Part print with two shaded views. Sizes in mm from the minimum x, y, z corner. A direction names the side the tool comes from. Give positions to 0.01 mm unless a question says otherwise; leave off trailing zeros. Order: outer loops, then holes, each group sorted by start corner. A loop starts at its lowest first (then second) coordinate and runs counter-clockwise, first axis right, second up. Notation, with made-up numbers: M 1.5,31.5 L 20.5,31.5 A16 ccw 20.5,62.5 Z; hole C 47,41.25 d4. An arc over 180 degrees is marked long. Answer as CSV lines item,"result".
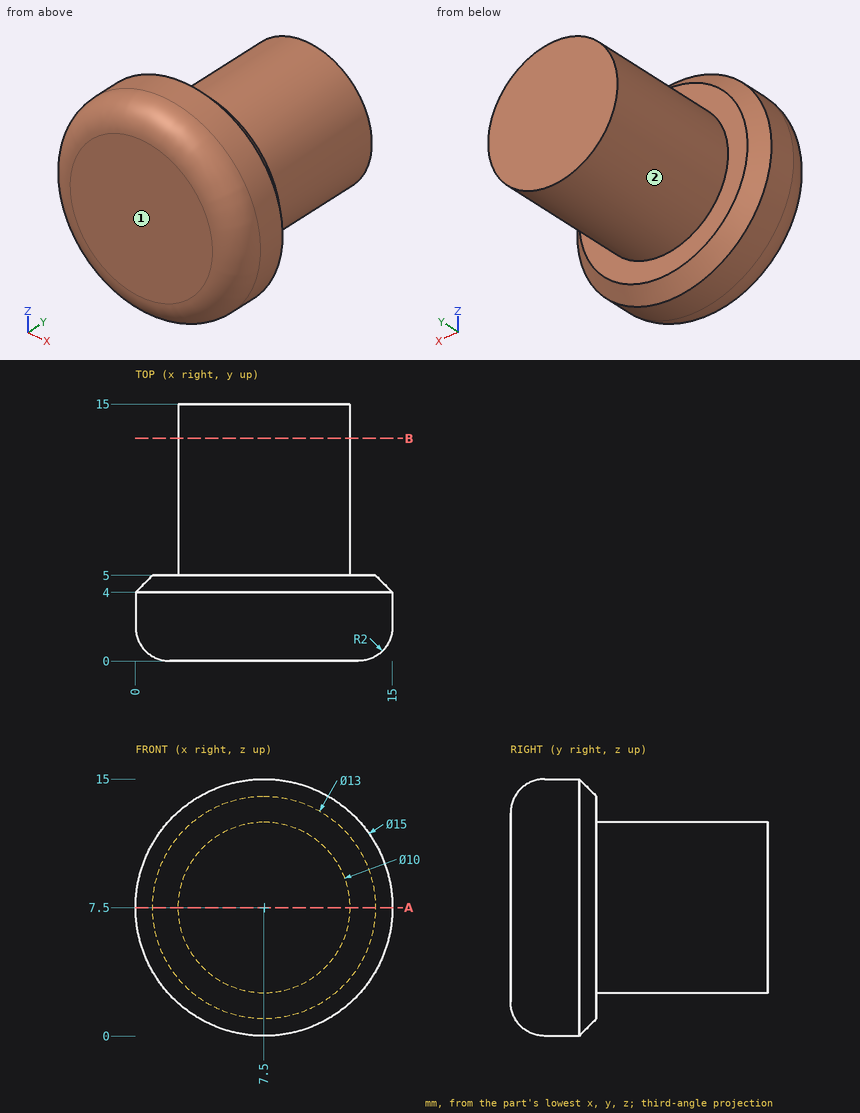
Item 1: Drop flat-ended pins along their axis: pin 1 (1.5 mm diameter, centred on x = 11.5, z = 2, fed in from -Y); pin 2 (5 mm diameter, centred on x = 2, y = 2.5, fed in from +Z); pin 3 (3 mm diameter, centred on x = 13, y = 10, fed in from -Z). Give the stop position or say it passes through.
Geometry says:
pin 1,"stops at y = 0.08"
pin 2,"stops at z = 14.37"
pin 3,"stops at z = 4.5"
Item 2: Band-saw the part on A-A (z = 7.5). Give the cut face in (x, y).
Geometry says:
outline,"M 0,2 A2 ccw 2,0 L 13,0 A2 ccw 15,2 L 15,4 L 14,5 L 12.5,5 L 12.5,15 L 2.5,15 L 2.5,5 L 1,5 L 0,4 Z"
Item 3: 3-axis set-ups, long thin cutter, end or side, ignore diameter. For the marked faces 1 and 2: which of +Z, -Z, +X, -X, +Y, -Y reach the whole face in a straight line?
Geometry says:
face 1,"+Z, -Z, +X, -X, -Y"
face 2,"+Y"
Item 4: Band-saw the part on B-B (y = 13). Give the cut face in (x, z), and give its area (3 significant figures).
Geometry says:
outline,"C 7.5,7.5 d10"
area,"78.5 mm2"
Item 5: Probe line 1 along Z through (x, y) = (9, 8.75); line 2 along X through (y, z) = (9, 7.75); line 3 along Z through (x, y) = (4.5, 12). List the from-to ranges inside material, lowest first. Write a range as from..to.
Geometry says:
line 1,"z = 2.73..12.27"
line 2,"x = 2.51..12.49"
line 3,"z = 3.5..11.5"
